from build123d import *

# Parameters (mm, degrees)
SKETCH_1_W           = 200
SKETCH_1_H           = 100
SKETCH_1_R           = 6.25
SKETCH_1_W_2         = 80
SKETCH_1_H_2         = 27
SKETCH_1_W_3         = 30
SKETCH_1_H_3         = 3.5
EXTRUDE_1_DEPTH      = 3
SKETCH_2_R           = 3
SKETCH_2_R_2         = 1.5
EXTRUDE_2_DEPTH      = 9
SKETCH_4_W           = 200
SKETCH_4_H           = 100
SKETCH_4_W_2         = 194
SKETCH_4_H_2         = 94
SKETCH_4_W_3         = 34
SKETCH_4_H_3         = 7.5
SKETCH_4_W_4         = 30
SKETCH_4_H_4         = 3.5
EXTRUDE_3_DEPTH      = 40
SKETCH_5_W           = 14
SKETCH_5_H           = 3.5
CUT_EXTRUDE_1_DEPTH  = 3
SKETCH_6_W           = 3
SKETCH_6_H           = 10
EXTRUDE_4_DEPTH      = 40
SKETCH_7_W           = 4.25
SKETCH_7_H           = 3.5
CUT_EXTRUDE_2_DEPTH  = 5
EXTRUDE_START        = 6.75
SKETCH_9_R           = 2.125
SKETCH_9_R_2         = 4.75
EXTRUDE_5_DEPTH      = 2
EXTRUDE_5_DEPTH_BACK = 1
SKETCH_10_R          = 3
SKETCH_10_R_2        = 1.5
EXTRUDE_6_DEPTH      = 5
SKETCH_11_R          = 1.5
SKETCH_11_R_2        = 0.5
EXTRUDE_7_DEPTH      = 5
EXTRUDE_START_2      = -3
EXTRUDE_8_DEPTH      = 1
FILLET_1_R           = 2


with BuildPart() as part:
    # Эскиз1 → Бобышка-Вытянуть1 (new body)
    with BuildSketch(Plane.XY):
        with Locations((40, 0)):
            Rectangle(SKETCH_1_W, SKETCH_1_H)
        with Locations((10, -25)):
            Circle(SKETCH_1_R, mode=Mode.SUBTRACT)
        with Locations((70, -25)):
            Circle(SKETCH_1_R, mode=Mode.SUBTRACT)
        with Locations((40, 13.5)):
            Rectangle(SKETCH_1_W_2, SKETCH_1_H_2, mode=Mode.SUBTRACT)
        with Locations((40, -25)):
            Rectangle(SKETCH_1_W_3, SKETCH_1_H_3, mode=Mode.SUBTRACT)
    extrude(amount=EXTRUDE_1_DEPTH)

    # Эскиз2 → Бобышка-Вытянуть2 (add)
    with BuildSketch(Plane(origin=(0, 0, 0), x_dir=(-1, 0, 0), z_dir=(0, 0, -1))):
        with Locations(Location((-86.625, 41, 0), (0, 0, 180))):
            Circle(SKETCH_2_R)
        with Locations((-86.625, 41)):
            Circle(SKETCH_2_R_2, mode=Mode.SUBTRACT)
        with Locations(Location((-86.625, -14, 0), (0, 0, 180))):
            Circle(SKETCH_2_R)
        with Locations(Location((-86.625, -14, 0), (0, 0, 180))):
            Circle(SKETCH_2_R_2, mode=Mode.SUBTRACT)
        with Locations(Location((6.625, -14, 0), (0, 0, 180))):
            Circle(SKETCH_2_R)
        with Locations((6.625, -14)):
            Circle(SKETCH_2_R_2, mode=Mode.SUBTRACT)
        with Locations(Location((6.625, 41, 0), (0, 0, 180))):
            Circle(SKETCH_2_R)
        with Locations(Location((6.625, 41, 0), (0, 0, 180))):
            Circle(SKETCH_2_R_2, mode=Mode.SUBTRACT)
    extrude(amount=EXTRUDE_2_DEPTH)

    # Эскиз4 → Бобышка-Вытянуть3 (add)
    with BuildSketch(Plane(origin=(0, 0, 0), x_dir=(-1, 0, 0), z_dir=(0, 0, -1))):
        with Locations((-40, 0)):
            Rectangle(SKETCH_4_W, SKETCH_4_H)
        with Locations((-40, 0)):
            Rectangle(SKETCH_4_W_2, SKETCH_4_H_2, mode=Mode.SUBTRACT)
        with Locations((-40, -25)):
            Rectangle(SKETCH_4_W_3, SKETCH_4_H_3)
        with Locations((-40, -25)):
            Rectangle(SKETCH_4_W_4, SKETCH_4_H_4, mode=Mode.SUBTRACT)
    extrude(amount=EXTRUDE_3_DEPTH)

    # Эскиз5 → Вырез-Вытянуть1 (cut)
    with BuildSketch(Plane.ZY.offset(-23)):
        with Locations((-31, -25)):
            Rectangle(SKETCH_5_W, SKETCH_5_H)
    extrude(amount=-CUT_EXTRUDE_1_DEPTH, mode=Mode.SUBTRACT)

    # Эскиз6 → Бобышка-Вытянуть4 (add)
    with BuildSketch(Plane(origin=(0, 0, 0), x_dir=(-1, 0, 0), z_dir=(0, 0, -1))):
        with Locations((23.5, -25)):
            Rectangle(SKETCH_6_W, SKETCH_6_H)
    extrude(amount=EXTRUDE_4_DEPTH)

    # Эскиз7 → Вырез-Вытянуть2 (cut)
    with BuildSketch(Plane.ZY.offset(25)):
        with Locations((-31.165446486, -25)):
            Rectangle(SKETCH_7_W, SKETCH_7_H)
    extrude(amount=-CUT_EXTRUDE_2_DEPTH, mode=Mode.SUBTRACT)

    # Эскиз9 → Бобышка-Вытянуть5 (add, two sides)
    with BuildSketch(Plane(origin=(0, -26.75, 0), x_dir=(1, 0, 0), z_dir=(0, 1, 0)).offset(EXTRUDE_START)) as extrude_5_sk:
        with BuildLine():
            Line((-31.538318399, 34.739296559), (-31.538318399, 0))
            Line((-31.538318399, 0), (-57, 0))
            Line((-57, 0), (-57, 34.739296559))
            Line((-57, 34.739296559), (-38.538318399, 34.739296559))
            ThreePointArc((-38.538318399, 34.739296559), (-37.513192133, 37.214170293), (-35.038318399, 38.239296559))
            ThreePointArc((-35.038318399, 38.239296559), (-32.563444665, 37.214170293), (-31.538318399, 34.739296559))
        make_face()
        with Locations(Location((-49.562204657, 3.1758428, 0), (0, 0, 90))):
            Circle(SKETCH_9_R, mode=Mode.SUBTRACT)
        with Locations(Location((-35.038318399, 34.739296559, 0), (0, 0, 90))):
            Circle(SKETCH_9_R, mode=Mode.SUBTRACT)
        with Locations(Location((-49, 22.040446486, 0), (0, 0, 90))):
            Circle(SKETCH_9_R_2, mode=Mode.SUBTRACT)
    extrude(amount=EXTRUDE_5_DEPTH)
    extrude(extrude_5_sk.sketch, amount=-EXTRUDE_5_DEPTH_BACK)

    # Эскиз10 → Бобышка-Вытянуть6 (add)
    with BuildSketch(Plane(origin=(0, 0, 0), x_dir=(-1, 0, 0), z_dir=(0, 0, -1))):
        with Locations(Location((50, 10, 0), (0, 0, 180))):
            Circle(SKETCH_10_R)
        with Locations((50, 10)):
            Circle(SKETCH_10_R_2, mode=Mode.SUBTRACT)
        with Locations(Location((23, 10, 0), (0, 0, 180))):
            Circle(SKETCH_10_R)
        with Locations((23, 10)):
            Circle(SKETCH_10_R_2, mode=Mode.SUBTRACT)
        with Locations(Location((23, 40, 0), (0, 0, 180))):
            Circle(SKETCH_10_R)
        with Locations((23, 40)):
            Circle(SKETCH_10_R_2, mode=Mode.SUBTRACT)
        with Locations(Location((50, 40, 0), (0, 0, 180))):
            Circle(SKETCH_10_R)
        with Locations((50, 40)):
            Circle(SKETCH_10_R_2, mode=Mode.SUBTRACT)
    extrude(amount=EXTRUDE_6_DEPTH)

    # Эскиз11 → Бобышка-Вытянуть7 (add)
    with BuildSketch(Plane(origin=(0, 0, 0), x_dir=(-1, 0, 0), z_dir=(0, 0, -1))):
        with Locations(Location((-120.5, 35.5, 0), (0, 0, 180))):
            Circle(SKETCH_11_R)
        with Locations((-120.5, 35.5)):
            Circle(SKETCH_11_R_2, mode=Mode.SUBTRACT)
        with Locations(Location((-105.15, 35.5, 0), (0, 0, 180))):
            Circle(SKETCH_11_R)
        with Locations((-105.15, 35.5)):
            Circle(SKETCH_11_R_2, mode=Mode.SUBTRACT)
        with Locations(Location((-105.15, -5.5, 0), (0, 0, 180))):
            Circle(SKETCH_11_R)
        with Locations((-105.15, -5.5)):
            Circle(SKETCH_11_R_2, mode=Mode.SUBTRACT)
        with Locations(Location((-120.5, -5.5, 0), (0, 0, 180))):
            Circle(SKETCH_11_R)
        with Locations((-120.5, -5.5)):
            Circle(SKETCH_11_R_2, mode=Mode.SUBTRACT)
    extrude(amount=EXTRUDE_7_DEPTH)

    # Эскиз12 → Бобышка-Вытянуть8 (add)
    with BuildSketch(Plane(origin=(0, 0, -40), x_dir=(-1, 0, 0), z_dir=(0, 0, -1)).offset(EXTRUDE_START_2)):
        with BuildLine():
            Line((-140, 40), (-140, 50))
            Line((-140, 50), (-130, 50))
            ThreePointArc((-130, 50), (-132.928932188, 42.928932188), (-140, 40))
        make_face()
        with BuildLine():
            Line((60, 40), (60, 50))
            Line((60, 50), (50, 50))
            ThreePointArc((50, 50), (52.928932188, 42.928932188), (60, 40))
        make_face()
        with BuildLine():
            Line((60, -50), (50, -50))
            ThreePointArc((50, -50), (52.928932188, -42.928932188), (60, -40))
            Line((60, -40), (60, -50))
        make_face()
        with BuildLine():
            Line((-140, -50), (-130, -50))
            ThreePointArc((-130, -50), (-132.928932188, -42.928932188), (-140, -40))
            Line((-140, -40), (-140, -50))
        make_face()
    extrude(amount=-EXTRUDE_8_DEPTH)

    # Скругление1
    fillet_1_edges = [part.edges().sort_by_distance(p)[0] for p in [
        (137, 43.730303993, -36),
        (133.730303993, 47, -36),
        (-57, 43.730303993, -36),
        (-53.730303993, 47, -36),
        (-57, -43.730303993, -36),
        (-53.730303993, -47, -36),
        (133.730303993, -47, -36),
        (137, -43.730303993, -36),
    ]]
    fillet(fillet_1_edges, radius=FILLET_1_R)


solid = part.part
Can you work these out from the model? Positions are in its coordinate system, mm. A direction names the side the tool comes from. Give positions to 0.01 mm unless a question says otherwise; leave off trailing zeros. Write each loop counter-clockwise with the first axis right and the second up, starting at its lowest first coordinate (ties: lowest second). Pieces come first, ordered by that corner, then holes. Notation, with made-up numbers: (52.25, -37.75) -> (101.25, -37.75) arc R12 cw to (101.25, -22.75) -> close; hole circle Ø6 at (-8.5, 60.25). An arc over 180 degrees is marked (long way). Answer as a JSON object with one key per item and string values. Group by question number.
Item 1: Suppose I cut it at B-B (x = 44). Please give me the cut outline in (y, z), plus the area to 4 significant figures.
Item 2: For faces 1 (the face through (40, -22, -40)), 2 (the face through (137, -1, -20)), 3 (the face through (-8, -13, -9)), which set-ups out of +Z, -Z, +X, -X, +Y, -Y let a thin tool reach every point of the face, with its end or its side?
Item 3: Suppose I cut it at C-C (y = 16). Please give me the cut outline in (x, z), plus the area to 3 significant figures.
Item 4: We'd pull the mould along X, two halves only. Please class faces 4 (the face through (40, 48, -40)), 5 (the face through (134, -44, -36)), 6 (the face through (-60, -1, -18)): +X half, -X half, draft (parallel to the pull), parting line (faces both ways), or undercut.
Item 5: Suppose I cut it at A-A (z = -14.5). Please give me the cut outline in (x, y), plus the area to 3 significant figures.
Item 6: I'm going to push flat-ended pins straight in: P1, Ø2, axis at x = 84, y = -14.5, coming from the -Z side; P2, Ø3, axis at x = -9, y = -21.5, coming from the -Z side; P3, Ø6.5, axis at x = -23, y = 39, coming from the -Z side. Where does each tip first touch, or does it pass through?
Item 7: Please list where these lines run through material, in increasing order: line 1 (X direction, y = -26, z = -11.5); line 2 (Y direction, x = 120.5, z = -1.5); line 3 (Y direction, x = 70, z = 1.15). Write a range as [from, to].
Item 8: Suppose I cut it at D-D (x = 101.5). Please give me the cut outline in (y, z).
Findings:
{
 "1": {"outline": "(-50, -40) -> (-47, -40) -> (-47, 0) -> (-28.75, 0) -> (-28.75, -40) -> (-26.75, -40) -> (-26.75, 3) -> (-50, 3) -> close; (-23.25, -40) -> (-21.25, -40) -> (-21.25, 0) -> (0, 0) -> (0, 3) -> (-23.25, 3) -> close; (27, 0) -> (47, 0) -> (47, -40) -> (50, -40) -> (50, 3) -> (27, 3) -> close", "area": "608.5 mm²"},
 "2": {"face 1": "-Z, +X, -X, +Y, -Y", "face 2": "none", "face 3": "-Z"},
 "3": {"outline": "(-60, -40) -> (-57, -40) -> (-57, 0) -> (0, 0) -> (0, 3) -> (-60, 3) -> close; (80, 0) -> (137, 0) -> (137, -40) -> (140, -40) -> (140, 3) -> (80, 3) -> close", "area": "600 mm²"},
 "4": {"face 4": "draft", "face 5": "undercut", "face 6": "-X half"},
 "5": {"outline": "(-60, -50) -> (140, -50) -> (140, 50) -> (-60, 50) -> close; (-25, -30) -> (-22, -30) -> (-22, -20) -> (-25, -20) -> close; (23, -28.75) -> (57, -28.75) -> (57, -21.25) -> (23, -21.25) -> close; hole (-57, -47) -> (137, -47) -> (137, 47) -> (-57, 47) -> (-57, -18) -> (-31.54, -18) -> (-31.54, -21) -> (-57, -21) -> close; hole (25, -26.75) -> (55, -26.75) -> (55, -23.25) -> (25, -23.25) -> close", "area": "2,020 mm²"},
 "6": {"P1": "stops at z = -9", "P2": "stops at z = 0", "P3": "stops at z = -5"},
 "7": {"line 1": "x = [-60, -57], [-25, -22], [23, 25], [55, 57], [137, 140]", "line 2": "y = [-50, -47], [-7, -6], [-5, -4], [34, 35], [36, 37], [47, 50]", "line 3": "y = [-50, -31.25], [-18.75, 0], [27, 50]"},
 "8": {"outline": "(-50, -40) -> (-47, -40) -> (-47, 0) -> (47, 0) -> (47, -40) -> (50, -40) -> (50, 3) -> (-50, 3) -> close"}
}
